The drawing under review shows one solid part. Ordinate dimensions are in mm from its lowest x, y, z. Give positions to 0.01 mm unless a question says otherwise; leave off trailing zeros. Loops run counter-clockwise (first coordinate to the right, second up) from the corner with the lowest first, then second, coordinate; pieces in that order, holes last. Notation, with made-up numbers: (43.5, 40) - (83.5, 40) arc R29 ccw to (83.5, 68) - close; hole circle Ø3 at (88, -34.5). An arc over 180 degrees is marked (long way). One line per item, written item: value. Start each with the question number.
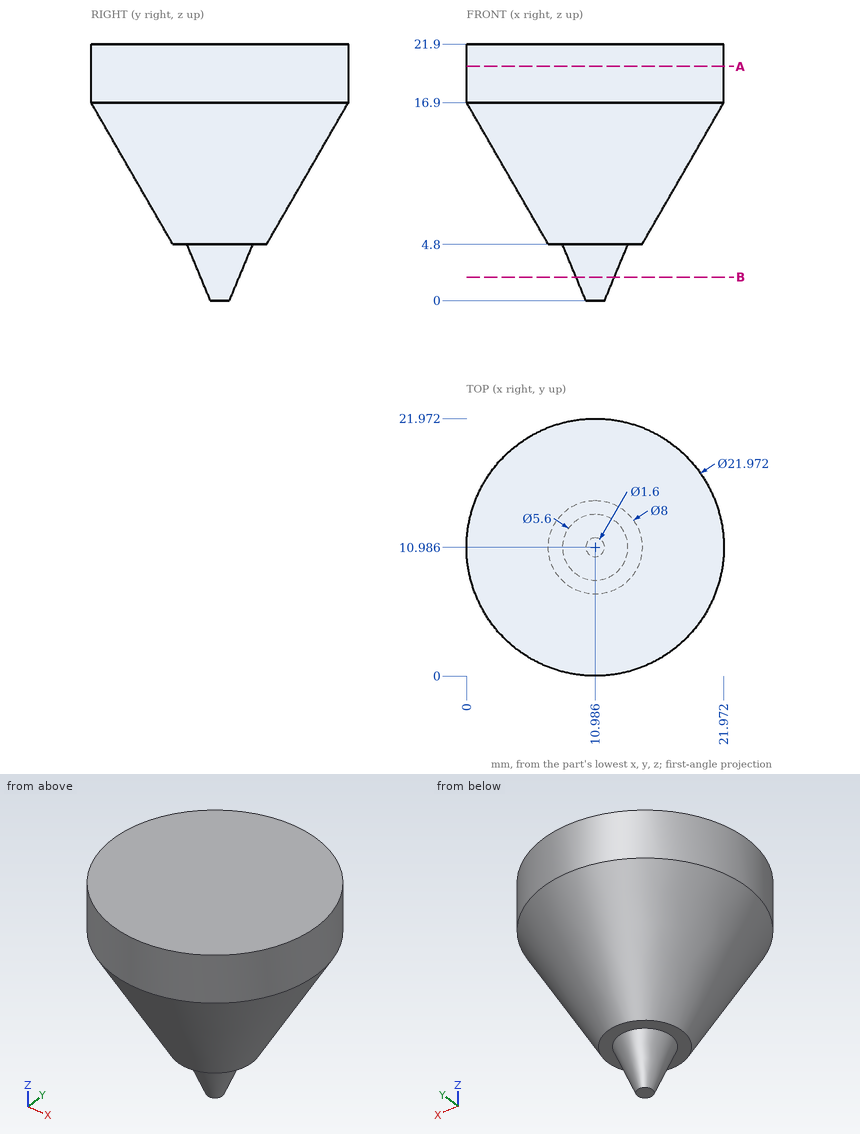
(1) Take a section at A-A on z = 20. State the section outline as (x, y) points, and give its area (3 significant figures).
(2) For pin 1 Ø1.5 at (x, y) = (11, 7.5) entering from -Z; pin 2 Ø1 at (x, y) = (10, 13.5) entering from -Z; pin 3 Ø8 at (y, z) = (19, 17) entering from -X, all flat-tipped, find the tip position at first contact; note any pin that passes through.
(3) Take a section at B-B on z = 2. State the section outline as (x, y) points, and give its area (3 significant figures).
(4) To check wall thickness, follow L1, parallel to X at y = 11, z = 21.25; L2, parallel to Z at x = 7.75, y = 7.5; L3, parallel to Y at x = 13, z = 7.5 (1 decimal). State the ranges of each line that lie inside material, in increasing order. Write a range as from..to.
Here are the results:
1. outline: circle Ø21.97 at (10.99, 10.99)
1. area: 379 mm²
2. pin 1: z = 4.65
2. pin 2: z = 3.36
2. pin 3: x = 0.76
3. outline: circle Ø3.27 at (10.99, 10.99)
3. area: 8.38 mm²
4. L1: 0..21.97
4. L2: 6.11..21.9
4. L3: 5.8..16.2
